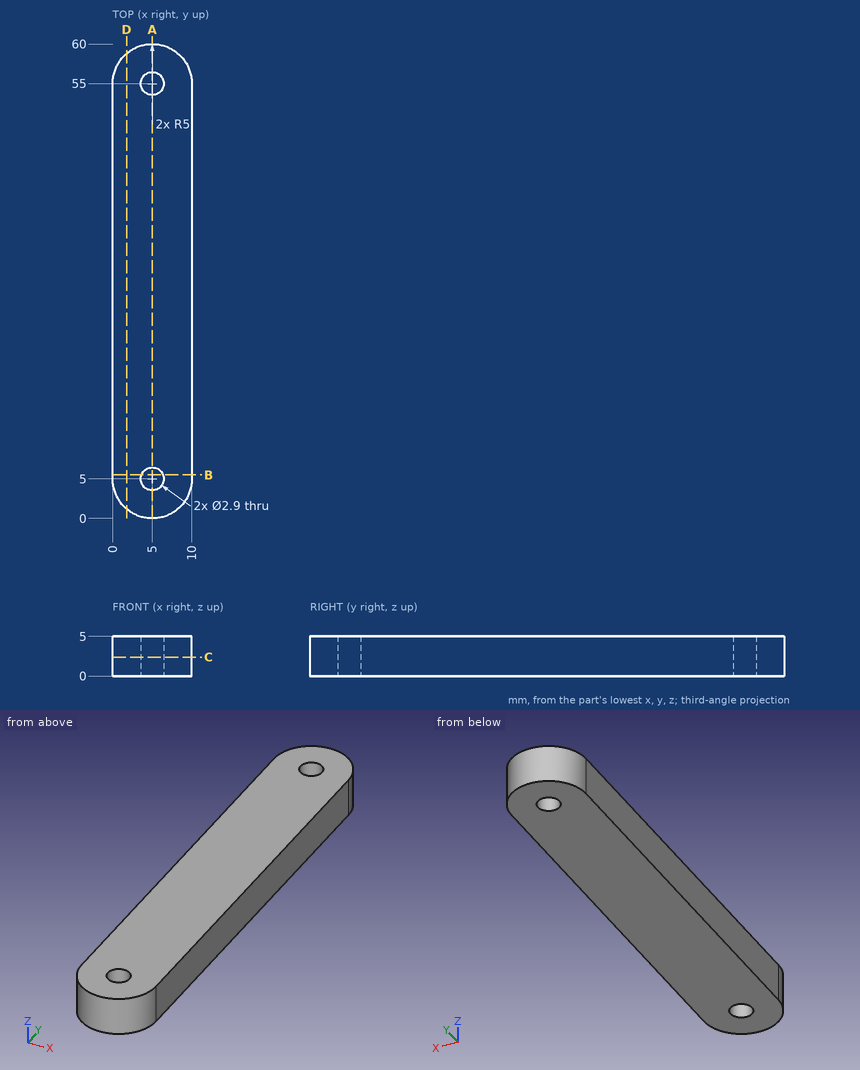
Design review of the part shown in the three views and the two pictorial views. Dimensions are in mm from the part's minimum x, y and z. Round coordinates to 2 decimals unless told otherwise and drop trailing zeros. Write each loop counter-clockwise with the first axis right and the second up, starting at its lowest first coordinate (ties: lowest second). Pieces come first, ordered by that corner, then holes. Notation, with made-up numbers: (2, 31) - (35, 31) arc R22 cw to (35, 49) - close; hole circle Ø4 at (-39, 85). An arc over 180 degrees is marked (long way). Answer as CSV lines item,"result". Start each with the question number.
(1) Add section C-C, the plane z = 2.4. State the section outline as (x, y) points, plus the area to 3 significant figures.
(2) Add section A-A, the plane x = 5. State the section outline as (y, z) points.
(3) For line 1 (Y direction, x = 5, z = 3.1); line 2 (Y direction, x = 5.75, z = 2); line 3 (Y direction, x = 3, z = 4.75), list the stretches that pass through material, from the lowest coordinate up.
(4) Add section B-B, the plane y = 5.5. State the section outline as (x, z) points, plus the area to 3 significant figures.
(5) Add section D-D, the plane x = 1.75. State the section outline as (y, z) points, plus the area to 3 significant figures.
From the geometry:
1,outline,"(0, 5) arc R5 ccw to (10, 5) - (10, 55) arc R5 ccw to (0, 55) - close; hole circle Ø2.9 at (5, 5); hole circle Ø2.9 at (5, 55)"
1,area,"565 mm²"
2,outline,"(0, 0) - (3.55, 0) - (3.55, 5) - (0, 5) - close; (6.45, 0) - (53.55, 0) - (53.55, 5) - (6.45, 5) - close; (56.45, 0) - (60, 0) - (60, 5) - (56.45, 5) - close"
3,line 1,"y = 0 to 3.55, 6.45 to 53.55, 56.45 to 60"
3,line 2,"y = 0.06 to 3.76, 6.24 to 53.76, 56.24 to 59.94"
3,line 3,"y = 0.42 to 59.58"
4,outline,"(0, 0) - (3.64, 0) - (3.64, 5) - (0, 5) - close; (6.36, 0) - (10, 0) - (10, 5) - (6.36, 5) - close"
4,area,"36.4 mm²"
5,outline,"(1.2, 0) - (58.8, 0) - (58.8, 5) - (1.2, 5) - close"
5,area,"288 mm²"
